Read the model definition and answer for the solid it produces. Units are mm, in the model's axes. A direction names the side the tool comes from. Give positions to 0.01 mm unless a question says otherwise; leave off trailing zeros. Order: outer loops, then holes, each group sorted by start corner. A loop starts at its lowest first (then second) coordinate and runs counter-clockwise, first axis right, second up.
```python
from build123d import *

# Parameters (mm, degrees)
SKETCH1_W           = 42
SKETCH1_H           = 42
BOSS_EXTRUDE1_DEPTH = 2
SKETCH2_W           = 0.5
SKETCH2_H           = 25
BOSS_EXTRUDE2_DEPTH = 2
SKETCH4_W           = 8.5
SKETCH4_H           = 27
BOSS_EXTRUDE3_DEPTH = 2
SKETCH5_W           = 5.42648105
SKETCH5_H           = 0.5
BOSS_EXTRUDE4_DEPTH = 15
SKETCH6_W           = 3.107576182
SKETCH6_H           = 27
BOSS_EXTRUDE5_DEPTH = 15
SKETCH7_W           = 2.5
SKETCH7_H           = 19
BOSS_EXTRUDE6_DEPTH = 10
SKETCH8_W           = 12
SKETCH8_H           = 5
SKETCH8_W_2         = 5
SKETCH8_H_2         = 10
BOSS_EXTRUDE7_DEPTH = 10
SKETCH9_R           = 2.25
SKETCH9_R_2         = 1.75
CUT_EXTRUDE1_DEPTH  = 1
SKETCH10_R          = 1.5
CUT_EXTRUDE2_DEPTH  = 3


with BuildPart() as part:
    # Sketch1 → Boss-Extrude1 (new body)
    with BuildSketch(Plane.XY):
        with Locations((35.471214637, -127.632705913)):
            Rectangle(SKETCH1_W, SKETCH1_H)
    extrude(amount=BOSS_EXTRUDE1_DEPTH)

    # Sketch2 → Boss-Extrude2 (add)
    with BuildSketch(Plane.XY.offset(2)):
        with Locations((19.721214637, -127.632705913)):
            Rectangle(SKETCH2_W, SKETCH2_H)
    extrude(amount=BOSS_EXTRUDE2_DEPTH)

    # Sketch4 → Boss-Extrude3 (add)
    with BuildSketch(Plane.XY.offset(4)):
        with Locations((20.721214637, -127.632705913)):
            Rectangle(SKETCH4_W, SKETCH4_H)
    extrude(amount=BOSS_EXTRUDE3_DEPTH)

    # Sketch5 → Boss-Extrude4 (add)
    with BuildSketch(Plane.XY.offset(6)):
        with Locations((21.665849022, -115.882705913)):
            Rectangle(SKETCH5_W, SKETCH5_H)
        with Locations((21.665849022, -120.382705913)):
            Rectangle(SKETCH5_W, SKETCH5_H)
        with Locations((21.665849022, -124.882705913)):
            Rectangle(SKETCH5_W, SKETCH5_H)
        with Locations((21.665849022, -130.382705913)):
            Rectangle(SKETCH5_W, SKETCH5_H)
        with Locations((21.665849022, -134.882705913)):
            Rectangle(SKETCH5_W, SKETCH5_H)
        with Locations((21.665849022, -139.382705913)):
            Rectangle(SKETCH5_W, SKETCH5_H)
    extrude(amount=BOSS_EXTRUDE4_DEPTH)

    # Sketch6 → Boss-Extrude5 (add)
    with BuildSketch(Plane.XY.offset(6)):
        with Locations((22.275002728, -127.632705913)):
            Rectangle(SKETCH6_W, SKETCH6_H)
    extrude(amount=BOSS_EXTRUDE5_DEPTH)

    # Sketch7 → Boss-Extrude6 (add)
    with BuildSketch(Plane.XY.offset(6)):
        with Locations((22.971214637, -127.632705913)):
            Rectangle(SKETCH7_W, SKETCH7_H)
    extrude(amount=BOSS_EXTRUDE6_DEPTH)

    # Sketch8 → Boss-Extrude7 (add)
    with BuildSketch(Plane.XY.offset(2)):
        with Locations((40.471214637, -110.132705913)):
            Rectangle(SKETCH8_W, SKETCH8_H)
        with Locations((40.471214637, -145.132705913)):
            Rectangle(SKETCH8_W, SKETCH8_H)
        with Locations((52.971214637, -127.632705913)):
            Rectangle(SKETCH8_W_2, SKETCH8_H_2)
    extrude(amount=BOSS_EXTRUDE7_DEPTH)

    # Sketch9 → Cut-Extrude1 (cut)
    with BuildSketch(Plane.XY.offset(12)):
        with Locations((37.471214637, -110.132705913)):
            Circle(SKETCH9_R)
        with Locations((43.471214637, -110.132705913)):
            Circle(SKETCH9_R)
        with Locations((52.971214637, -125.132705913)):
            Circle(SKETCH9_R_2)
        with Locations((52.971214637, -130.132705913)):
            Circle(SKETCH9_R_2)
        with Locations((43.471214637, -145.132705913)):
            Circle(SKETCH9_R)
        with Locations((37.471214637, -145.132705913)):
            Circle(SKETCH9_R)
    extrude(amount=-CUT_EXTRUDE1_DEPTH, mode=Mode.SUBTRACT)

    # Sketch10 → Cut-Extrude2 (cut, through all)
    with BuildSketch(Plane.XY.offset(2)):
        with Locations((53.971214637, -109.132705913)):
            Circle(SKETCH10_R)
        with Locations((16.971214637, -109.132705913)):
            Circle(SKETCH10_R)
        with Locations((16.971214637, -146.132705913)):
            Circle(SKETCH10_R)
        with Locations((53.971214637, -146.132705913)):
            Circle(SKETCH10_R)
    extrude(amount=-CUT_EXTRUDE2_DEPTH, mode=Mode.SUBTRACT)


solid = part.part
```
1) The part is cut by section B-B on x = 37. Determine the outline of the cut face in (y, z).
Final values:
outline: (-148.63, 0) - (-106.63, 0) - (-106.63, 2) - (-107.63, 2) - (-107.63, 12) - (-107.93, 12) - (-107.93, 11) - (-112.33, 11) - (-112.33, 12) - (-112.63, 12) - (-112.63, 2) - (-142.63, 2) - (-142.63, 12) - (-142.93, 12) - (-142.93, 11) - (-147.33, 11) - (-147.33, 12) - (-147.63, 12) - (-147.63, 2) - (-148.63, 2) - close
2) A tool of negligible diameter and unlimited length cuts with its end or side. For faces 4 (the face through (20.721, -140, 13)), 5 (the face through (52.59, -131.84, 11.51)), 6 (the face through (22, -141.133, 10)), from which of +Z, -Z, +X, -X, +Y, -Y can it reach the whole face along a straight path? Write none if from no direction.
Final values:
face 4: +Z, -X, -Y
face 5: +Z
face 6: +Z, +X, -X, -Y
3) Consider L1, parallel to Y at x = 20, z = 20; L2, parallel to Y at x = 46, z = 8.5; L3, parallel to X at y = -145, z = 11.5. Determine where each line is inside the solid, lowest interval first.
Final values:
L1: y = -139.63 to -139.13, -135.13 to -134.63, -130.63 to -130.13, -125.13 to -124.63, -120.63 to -120.13, -116.13 to -115.63
L2: y = -147.63 to -142.63, -112.63 to -107.63
L3: x = 34.47 to 35.23, 39.72 to 41.23, 45.72 to 46.47
4) The part is cut by section A-A on y = -117.5. Determine the outline of the cut face in (x, z), and give its area (3 significant figures).
Final values:
outline: (14.47, 0) - (56.47, 0) - (56.47, 2) - (19.97, 2) - (19.97, 4) - (24.97, 4) - (24.97, 6) - (23.83, 6) - (23.83, 21) - (20.72, 21) - (20.72, 6) - (16.47, 6) - (16.47, 4) - (19.47, 4) - (19.47, 2) - (14.47, 2) - close
area: 149 mm2
5) The part is cut by section D-D on y = -111.5. Determine the outline of the cut face in (x, z), and give its area (3 significant figures).
Final values:
outline: (14.47, 0) - (56.47, 0) - (56.47, 2) - (46.47, 2) - (46.47, 12) - (45.26, 12) - (45.26, 11) - (41.68, 11) - (41.68, 12) - (39.26, 12) - (39.26, 11) - (35.68, 11) - (35.68, 12) - (34.47, 12) - (34.47, 2) - (14.47, 2) - close
area: 197 mm2
6) For a pull along X with two mould halves and no side action, classify faces 1 (the face through (46.471, -110, 7)), 2 (the face through (40, -147.633, 7)), 3 (the face through (43, -110, 11)) as released by +X, released by -X, zero draft, split by the parting line, or undercut.
Final values:
face 1: released by +X
face 2: zero draft
face 3: undercut
7) Given pin 1 (4 mm diameter, centred on x = 37.47, y = -110.13, fed in from +Z); pin 2 (1.5 mm diameter, centred on x = 54, z = 7, fed in from +Y); pin 3 (2 mm diameter, centred on y = -119.5, z = 11, fed in from +X), each flat-ended and moving along its own axis, determine where each tip first touches the part or whether it passes through.
Final values:
pin 1: stops at z = 11
pin 2: stops at y = -122.63
pin 3: stops at x = 24.38
8) The part is cut by section C-C on z = 10.25. Count the separate pieces of the cut face and the enclosed holes in it, and give its area (3 significant figures).
Final values:
separate pieces: 4
enclosed holes: 0
area: 268 mm2
